Work out the finished part from the listing and answer in its coordinate system (mm). A direction names the side the tool comes from. Round coordinates to 2 decimals unless told otherwise and drop trailing zeros. Loops run counter-clockwise (first coordinate to the right, second up) from the corner with the lowest first, then second, coordinate; pieces in that order, holes last. Notation, with made-up numbers: (-21, -15.5) - (-14, -15.5) arc R21 ccw to (-14, -0.5) - close; hole circle Ø5 at (70.5, 0). An arc over 180 degrees is marked (long way). Return JSON: item names as keys, results as strings.
from build123d import *

# Parameters (mm, degrees)
EXTRUDE_1_OUTLINE_R = 4.5
EXTRUDE_1_DEPTH     = 7.5
FILLET_1_R          = 2
FILLET_2_R          = 1
CHAMFER_1_SIZE      = 3


# Read off the part's stored shape, not the designer's step: 伸長1
with BuildPart() as part:
    # 伸長1 outline → 伸長1 (new body)
    with BuildSketch(Plane(origin=(0, 0, 0), x_dir=(1, 0, 0), z_dir=(0, 1, 0))):
        with BuildLine():
            ThreePointArc((18.33030278, 8), (0, 20), (-18.33030278, 8))
            Line((-18.33030278, 8), (-22.5, 8))
            ThreePointArc((-22.5, 8), (-30.5, 0), (-22.5, -8))
            Line((-22.5, -8), (-18.33030278, -8))
            ThreePointArc((-18.33030278, -8), (0, -20), (18.33030278, -8))
            Line((18.33030278, -8), (22.5, -8))
            ThreePointArc((22.5, -8), (30.5, 0), (22.5, 8))
            Line((22.5, 8), (18.33030278, 8))
        make_face()
        with Locations((-22.5, 0)):
            Circle(EXTRUDE_1_OUTLINE_R, mode=Mode.SUBTRACT)
        with Locations((22.5, 0)):
            Circle(EXTRUDE_1_OUTLINE_R, mode=Mode.SUBTRACT)
    extrude(amount=EXTRUDE_1_DEPTH)

    # 圓角1
    fillet_1_edges = [part.edges().sort_by_distance(p)[0] for p in [
        (18.33030278, 3.75, -8),
        (18.33030278, 3.75, 8),
        (-18.33030278, 3.75, 8),
        (-18.33030278, 3.75, -8),
    ]]
    fillet(fillet_1_edges, radius=FILLET_1_R)

    # 草圖3 → 旋轉1 (revolve)
    with BuildSketch(Plane.XY, mode=Mode.PRIVATE) as revolve_1_sk:
        Polygon((0, 25.5), (12.5, 25.5), (15, 7.5), (0, 7.5), align=None)
    revolve(revolve_1_sk.sketch.rotate(Axis((0, 0, 0), (0, 1, 0)), 90), axis=Axis((0, 0, 0), (0, 1, 0)))

    # 圓角2
    fillet_2_edges = [part.edges().sort_by_distance(p)[0] for p in [
        (-30.5, 7.5, 0),
        (-21.047958971, 7.5, 8),
        (30.5, 7.5, 0),
        (21.047958971, 7.5, -8),
        (21.047958971, 7.5, 8),
        (0, 7.5, 20),
        (0, 7.5, -20),
        (-21.047958971, 7.5, -8),
        (18.551452007, 7.5, 8.294394269),
        (18.551452007, 7.5, -8.294394269),
        (-18.551452007, 7.5, -8.294394269),
        (-18.551452007, 7.5, 8.294394269),
        (0, 7.5, 15),
    ]]
    fillet(fillet_2_edges, radius=FILLET_2_R)

    # 草圖4 → 除料-旋轉1 (revolve, cut)
    with BuildSketch(Plane.XY, mode=Mode.PRIVATE) as cut_revolve_1_sk:
        Polygon((0, 0), (4.5, 0), (4.5, 7.5), (10.5, 7.5), (10.5, 10.5), (0, 10.5), align=None)
    revolve(cut_revolve_1_sk.sketch.rotate(Axis((0, 0, 0), (0, 1, 0)), 90), axis=Axis((0, 0, 0), (0, 1, 0)), mode=Mode.SUBTRACT)

    # 導角1
    chamfer_1_edges = [part.edges().sort_by_distance(p)[0] for p in [
        (0, 0, 4.5),
    ]]
    chamfer(chamfer_1_edges, length=CHAMFER_1_SIZE)

    # 草圖7 → 3/8 Rc 螺紋孔1 (revolve, cut)
    with BuildSketch(Plane(origin=(0, 25.5, 0), x_dir=(0, 0, 1), z_dir=(1, 0, 0))):
        Polygon((0, 0), (0, 22.386153426), (7.15, 18.09), (7.15, 11.4), (7.54713052, 11.4), (7.903, 0), align=None)
    revolve(axis=Axis((0, 31.85, 0), (0, -1, 0)), mode=Mode.SUBTRACT)


solid = part.part
1) Section D-D (y = 23.5) is taken. Give the vertices of the cut face in (x, z).
Verdict:
{"outline": "circle Ø25.56 at (0, 0); hole circle Ø15.68 at (0, 0)"}
2) Section C-C (z = -2) is taken. Count the separate pieces of the cut face and the enclosed holes in it, and give its area (3 significant figures).
Verdict:
{"separate pieces": "4", "enclosed holes": "0", "area": "466 mm2"}
3) A tool of negligible diameter and unlimited length cuts with its end or side. For faces 1 (the cylindrical face through (18.56, 3.3, 8.29)), 2 (the cylindrical face through (-27, 4, 0)), 3 (the flat face through (6.9, 10.5, 2.5)), 4 (the cylindrical face through (-7.09, 12.33, -0.93)), 5 (the flat face through (-21, 3, 8)), from which of +Z, -Z, +X, -X, +Y, -Y can it reach the whole face along a straight path? Write none if from no direction.
Verdict:
{"face 1": "+Z, +X, +Y, -Y", "face 2": "+Y, -Y", "face 3": "none", "face 4": "+Y", "face 5": "+Z, -X, +Y, -Y"}
4) Section B-B (y = 16.75) is taken. Give the vertices of the cut face in (x, z).
Verdict:
{"outline": "circle Ø27.43 at (0, 0); hole circle Ø15.26 at (0, 0)"}
5) Find the intervals of material crossed by L1, parallel to X at y = 3.5, z = 0; L2, parallel to Y at x = -4, z = -7; L3, parallel to Z at x = -22.5, y = 3, in increasing order.
Verdict:
{"L1": "x = -30.5 to -27, -18 to -4.5, 4.5 to 18, 27 to 30.5", "L2": "y = 0 to 7.5, 10.5 to 25.5", "L3": "z = -8 to -4.5, 4.5 to 8"}
6) Determine the mould class of faces 6 (the flat face through (21, 3, 8)), 7 (the cylindrical face through (18, 4, 0)), 8 (the conical face through (11.926, 18.715, -6.203)) for opening direction Z: pulls with the +Z half, pulls with the -Z half, needs draft (parallel to the pull), parting line crosses it, or undercut.
Verdict:
{"face 6": "pulls with the +Z half", "face 7": "undercut", "face 8": "parting line crosses it"}
7) Flat-ended cylindrical pins translate along their axes: pin 1 (13 mm diameter, centred on x = 0, z = 0, fed in from +Y); pin 2 (7 mm diameter, centred on x = -22.5, z = 0, fed in from +Y); pin 3 (6 mm diameter, centred on x = -13.5, y = 13, fed in from +Z); pin 4 (4 mm diameter, centred on x = -2, y = 10, fed in from -Z). Find the tip coordinate at first contact, or state that the pin passes through.
Verdict:
{"pin 1": "stops at y = 7.02", "pin 2": "passes through", "pin 3": "stops at z = 9.67", "pin 4": "stops at z = -14.9"}
